Geometry: final body of the model. Coordinates: model frame, mm. Face numbers are marked on the shaded views. A direction names the side the tool comes from. Coordinates: 2 decimals unless noted, no trailing zeros. Order: outer loops, then holes, each group sorted by start corner. A loop starts at its lowest first (then second) coordinate and runs counter-clockwise, first axis right, second up. Notation, with made-up numbers: (-13, -7) -> (-2, -7) arc R10 cw to (-2, -2) -> close; hole circle Ø6 at (-19.5, 52.5). An arc over 180 degrees is marked (long way). Use one line per item in the form item = value.
```python
from build123d import *

# Parameters (mm, degrees)
F0_W     = 106.147542
F0_H     = 54.795082
F1_DEPTH = 7.5
F2_W     = 81.475418
F2_H     = 41.885248
F3_DEPTH = 133.7


with BuildPart() as f1:
    # F0 (on Top) → F1 (new body, symmetric)
    with BuildSketch(Plane.XY):
        with Locations((-4.877049, 0)):
            Rectangle(F0_W, F0_H)
    extrude(amount=F1_DEPTH, both=True)

    # F2 (on face) → F3 (join)
    with BuildSketch(Plane.XY.offset(7.5)):
        with Locations((-12.336066, 3.012295)):
            Rectangle(F2_W, F2_H)
    extrude(amount=F3_DEPTH)


solid = f1.part
```
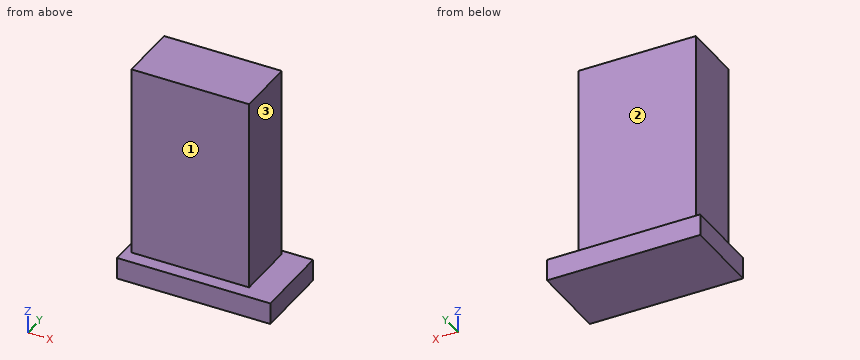
1) Access query for the marked faces 1, 2 and 3. Directions: +Z, -Z, +X, -X, +Y, -Y. A direction counts if a zero-diameter tool reaches every point of the face in a straight line with its end or side. Return the directions, or none.
Results found:
face_1 = +Z, +X, -X, -Y
face_2 = +Z, +X, -X, +Y
face_3 = +Z, +X, +Y, -Y
2) Contact query for flat-ended pins moving along their axis: P1, Ø21, axis at y = -4, z = 71, coming from the -X side; P2, Ø1, axis at x = -29.5, z = 105.5, coming from the +Y side; P3, Ø12.5, axis at y = 7, z = 42, coming from the +X side. Output: stop coordinate, or through.
Results found:
P1 = -53.07
P2 = 23.95
P3 = 28.4
3) Section C-C, the plane z = 94. Output: boundary loops of the cut face in (x, y).
Results found:
outline = (-53.07, -17.93) -> (28.4, -17.93) -> (28.4, 23.95) -> (-53.07, 23.95) -> close
4) Material intervals for probe 1 along Z at (x, y) = (-11.5, 24); probe 2 along Y at (x, z) = (-40.5, 109.5); probe 3 along X at (y, z) = (9, 86.5), sorted ascending. Write a range as from..to.
Results found:
probe_1 = -7.5..7.5
probe_2 = -17.93..23.95
probe_3 = -53.07..28.4
5) Section D-D, the plane x = 30. Output: boundary loops of the cut face in (y, z), and give its area (3 significant figures).
Results found:
outline = (-27.4, -7.5) -> (27.4, -7.5) -> (27.4, 7.5) -> (-27.4, 7.5) -> close
area = 822 mm2
6) Section A-A, the plane x = -18. Output: boundary loops of the cut face in (y, z).
Results found:
outline = (-27.4, -7.5) -> (27.4, -7.5) -> (27.4, 7.5) -> (23.95, 7.5) -> (23.95, 141.2) -> (-17.93, 141.2) -> (-17.93, 7.5) -> (-27.4, 7.5) -> close
7) Section B-B, the plane y = -12.5. Output: boundary loops of the cut face in (x, z).
Results found:
outline = (-57.95, -7.5) -> (48.2, -7.5) -> (48.2, 7.5) -> (28.4, 7.5) -> (28.4, 141.2) -> (-53.07, 141.2) -> (-53.07, 7.5) -> (-57.95, 7.5) -> close
